Job drawing, mm, ordinate dimensions from the low corner. One solid piece. Round coordinates to 2 decimals unless told otherwise and drop trailing zeros. Write each loop counter-clockwise with the first axis right and the second up, starting at its lowest first coordinate (ties: lowest second). Pieces come first, ordered by that corner, then holes. Notation, with made-up numbers: (65, -21) - (81, -21) arc R23 cw to (81, -7) - close; hole circle Ø11 at (35.25, 29). An arc over 180 degrees is marked (long way). Write each question's results on one line, items separated by ' | '.
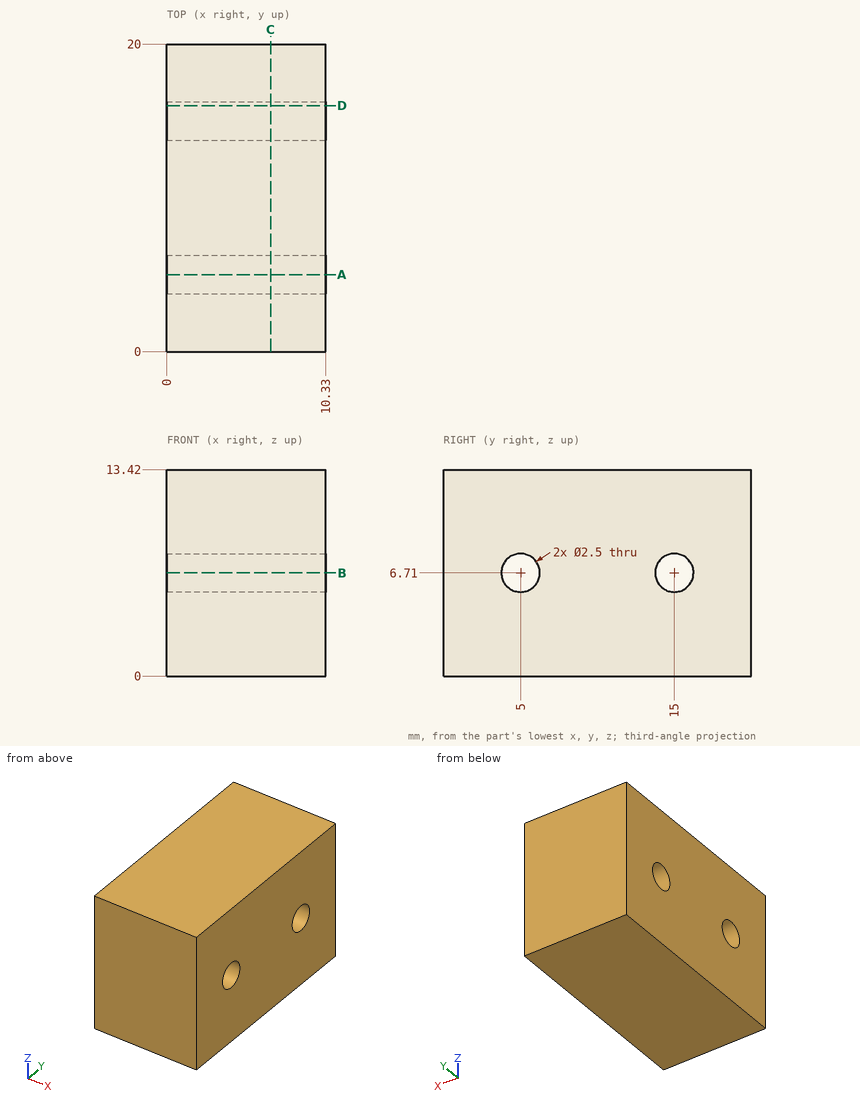
(1) Drill centre lines: probe 1 along Y at (x, z) = (4.75, 6.71); probe 2 along Z at (x, y) = (4, 15.75); probe 3 along Z at (x, y) = (3.5, 14.75). Where is each one in solid material? Low to high. Write a range as [from, to].
Worked answers:
probe 1: y = [0, 3.75], [6.25, 13.75], [16.25, 20] | probe 2: z = [0, 5.71], [7.71, 13.42] | probe 3: z = [0, 5.49], [7.93, 13.42]
(2) Slice it at D-D, the plane y = 16. Write the cut outline in (x, z).
Worked answers:
outline: (0, 0) - (10.33, 0) - (10.33, 5.96) - (0, 5.96) - close; (0, 7.46) - (10.33, 7.46) - (10.33, 13.42) - (0, 13.42) - close
(3) Slice it at B-B, the plane z = 6.71. Write the cut outline in (x, y).
Worked answers:
outline: (0, 0) - (10.33, 0) - (10.33, 3.75) - (0, 3.75) - close; (0, 6.25) - (10.33, 6.25) - (10.33, 13.75) - (0, 13.75) - close; (0, 16.25) - (10.33, 16.25) - (10.33, 20) - (0, 20) - close
(4) Slice it at A-A, the plane y = 5. Write the cut outline in (x, z), and give its area (3 significant figures).
Worked answers:
outline: (0, 0) - (10.33, 0) - (10.33, 5.46) - (0, 5.46) - close; (0, 7.96) - (10.33, 7.96) - (10.33, 13.42) - (0, 13.42) - close | area: 113 mm2
(5) Slice it at C-C, the plane x = 6.75. Write the cut outline in (y, z).
Worked answers:
outline: (0, 0) - (20, 0) - (20, 13.42) - (0, 13.42) - close; hole circle Ø2.5 at (5, 6.71); hole circle Ø2.5 at (15, 6.71)
